For this review, take the finished solid that the model builds, in its own axes (mm). A direction names the side the tool comes from. Give positions to 0.01 mm unless a question says otherwise; leave off trailing zeros. Write each loop counter-clockwise with the first axis right and the second up, starting at its lowest first coordinate (ties: lowest second). Pieces come first, ordered by that corner, then holes. Notation, with made-up numbers: M 79,41.5 L 101,41.5 A15 ccw 101,50.5 Z; hole C 80.5,-10 d9. An arc over 180 degrees is marked long. One line per item, written item: value. Start each with the question number.
Item 1: Consider section B-B, the plane y = 6.5. Write out the cut boundary in (x, z).
Item 2: Consider section C-C, the plane z = 36.5. Write out the cut boundary in (x, y).
Item 3: Tool access review of faces 1 (the face through (16, 31, -8)), 2 (the face through (-7.5, 173.2, 34.9)): name each direction out of +Z, -Z, +X, -X, +Y, -Y from which nothing blocks a thin tool from reaching the whole face with its end or side.
Item 4: To check wall thickness, follow probe 1 along X at (y, z) = (141.5, 38); probe 2 along X at (y, z) = (202.5, 86); probe 3 along Z at (x, y) = (-10, 141.5). State the ranges of each line that lie inside material, in increasing order.
Item 5: Consider section D-D, the plane y = -64. Write out the cut boundary in (x, z), and give its area (3 significant figures).
Item 6: Consider section A-A, the plane x = 7.5. Write out the cut boundary in (y, z) (3 decimals).
Item 7: Mouldability with a two-part tool opening along Z and no side actions: class faces 3 (the face through (-11, 86, 36)), 4 (the face through (7.5, 173.2, 34.9)), 5 (the face through (0.15, 9.69, 35.76)) as released by +Z, released by -Z, zero draft, split by the parting line, or undercut.
Item 8: Clearance check with flat-ended pins moving along their axes: pin 1 Ø3 at (x, y) = (-6, -17) entering from -Z; pin 2 Ø6 at (x, z) = (2, 51.5) entering from +Y; pin 3 Ø6 at (x, y) = (-10, 67.5) entering from +Z. State where each tip first meets the part, or that it passes through.
```python
from build123d import *

# Parameters (mm, degrees)
F2_DEPTH = 16
F3_DEPTH = 4
F4_DEPTH = 11


with BuildPart() as f2:
    # F1 (on Right) → F2 (new body, symmetric)
    with BuildSketch(Plane.YZ):
        with BuildLine():
            Line((150.3560738462, 25), (0, 25))
            ThreePointArc((0, 25), (-75.426387367, 19.4523172703), (-149.2294073105, 2.9286693037))
            Line((-149.2294073105, 2.9286693037), (-149.2294073105, 0))
            Line((-149.2294073105, 0), (-149.2294073105, -27.0713306963))
            ThreePointArc((-149.2294073105, -27.0713306963), (-48.6487574396, -41.4344679398), (52.6726568851, -33.9020155382))
            Line((52.6726568851, -33.9020155382), (209.5149365225, -5))
            Line((209.5149365225, -5), (215.8916333726, 25))
            Line((215.8916333726, 25), (171.0938662291, 25))
            Line((171.0938662291, 25), (150.3560738462, 25))
        make_face()
    extrude(amount=F2_DEPTH, both=True)

    # F1 (on Right) → F3 (join, symmetric)
    with BuildSketch(Plane.YZ):
        Polygon((175.3449974625, 45), (171.0938662291, 25), (215.8916333726, 25), (230.7705926895, 95), (190.7705926895, 95), (162.4827761164, 46.0040644602), align=None)
    extrude(amount=F3_DEPTH, both=True)

    # F1 (on Right) → F4 (join, symmetric)
    with BuildSketch(Plane.YZ):
        Polygon((162.4827761164, 46.0040644602), (150.3560738462, 25), (171.0938662291, 25), (175.3449974625, 45), align=None)
        with BuildLine():
            Line((19.114555791, 46.2288648769), (0, 25))
            Line((0, 25), (150.3560738462, 25))
            Line((150.3560738462, 25), (162.4827761164, 46.0040644602))
            Line((162.4827761164, 46.0040644602), (72.8637576103, 53))
            ThreePointArc((72.8637576103, 53), (45.6439579452, 52.3546166529), (19.114555791, 46.2288648769))
        make_face()
    extrude(amount=F4_DEPTH, both=True)


solid = f2.part
```
Model answer:
1. outline: M -16,-40.07 L 16,-40.07 L 16,25 L 11,25 L 11,32.22 L -11,32.22 L -11,25 L -16,25 Z
2. outline: M -11,10.35 L 11,10.35 L 11,173.54 L 4,173.54 L 4,218.34 L -4,218.34 L -4,173.54 L -11,173.54 Z
3. face 1: +Z, -Z, +X, +Y, -Y
3. face 2: -X, +Y
4. probe 1: x = -11 to 11
4. probe 2: x = -4 to 4
4. probe 3: z = -17.53 to 47.64
5. outline: M -16,-40.66 L 16,-40.66 L 16,21.01 L -16,21.01 Z
5. area: 1,970 mm2
6. outline: M -149.229,-27.071 A471.185 ccw 52.673,-33.902 L 209.515,-5 L 215.892,25 L 171.094,25 L 175.345,45 L 72.864,53 A134.21 ccw 19.115,46.229 L 0,25 A515.523 ccw -149.229,2.929 Z
7. face 3: zero draft
7. face 4: undercut
7. face 5: released by +Z
8. pin 1: stops at z = -41.49
8. pin 2: stops at y = 222.16
8. pin 3: stops at z = 53.39
